Source: CAD feature listing. Evaluate the final solid. Frame: model axes, mm. Coordinates: 2 decimals unless noted, no trailing zeros. Write each loop counter-clockwise with the first axis right and the second up, starting at its lowest first coordinate (ties: lowest second). Pieces come first, ordered by that corner, then holes. Notation, with made-up numbers: (72.5, 70.25) -> (86.5, 70.25) arc R20 cw to (86.5, 109.25) -> close; hole circle Ø4 at (-15, 33.25). An arc over 180 degrees is marked (long way). Write item = value, one per line.
from build123d import *

# Parameters (mm, degrees)
F4_R     = 10.2299469816
F0_DEPTH = 127
F1_R     = 13.3830980952
F5_DEPTH = 25.4
F3_SIZE  = 10.16
F6_R     = 5.08


# Not quite as in the source:
# - a fillet or chamfer that OpenCascade refuses, or shapes differently, is made with other operations: its cross-section is extruded or revolved along the edge and cut away or added


with BuildPart() as f0:
    # F4 (on Top) → F0 (new body)
    with BuildSketch(Plane.XY):
        Circle(F4_R)
    extrude(amount=F0_DEPTH)

    # F1 (on face) → F5 (join)
    with BuildSketch(Plane.XY.offset(127)):
        Circle(F1_R)
    extrude(amount=F5_DEPTH)

    # F2: fillet of radius 5.08 on 1 edges, made by hand

    # F2_s1 → F2_t2 (revolve, cut)
    with BuildSketch(Plane.XZ):
        with BuildLine():
            ThreePointArc((13.3830980952, 131.7003886402), (12.5217941226, 128.870370296), (10.2299469816, 127))
            Line((10.2299469816, 127), (13.3830980952, 127))
            Line((13.3830980952, 127), (13.3830980952, 131.7003886402))
        make_face()
    revolve(axis=Axis((0, 0, 127), (0, 0, 1)), mode=Mode.SUBTRACT)

    # F3
    f3_edges = [f0.edges().sort_by_distance(p)[0] for p in [
        (-13.383098, 0, 152.4),
    ]]
    chamfer(f3_edges, length=F3_SIZE)

    # F6
    f6_edges = [f0.edges().sort_by_distance(p)[0] for p in [
        (-3.223098, 0, 152.4),
    ]]
    fillet(f6_edges, radius=F6_R)


solid = f0.part
1) Cut plane B-B, the plane z = 73. Output: boundary loops of the cut face in (x, y).
Answer block:
outline = circle Ø20.46 at (0, 0)
2) First-contact query: pin 1 Ø6 at (x, z) = (-4, 46) entering from +Y; pin 2 Ø3 at (x, z) = (-6.5, 16) entering from +Y; pin 3 Ø2 at (x, z) = (8, 73.5) entering from +Y; pin 4 Ø10 at (x, y) = (3.5, 5) entering from -Z. Flat tips, straight axial feed; report the tip coordinate or a pass-through.
Answer block:
pin_1 = 10.18
pin_2 = 8.92
pin_3 = 7.46
pin_4 = 0
3) Material intervals for probe 1 along Y at (x, z) = (-0.5, 50); probe 2 along Y at (x, z) = (-1.5, 72); probe 3 along X at (y, z) = (-7, 33.5), sorted ascending. Write a range as [from, to].
Answer block:
probe_1 = [-10.22, 10.22]
probe_2 = [-10.12, 10.12]
probe_3 = [-7.46, 7.46]
4) Cut plane A-A, the plane z = 136.5. Output: boundary loops of the cut face in (x, y), and give its area (3 significant figures).
Answer block:
outline = circle Ø26.77 at (0, 0)
area = 563 mm2
5) Pull-direction query (X, two-part tool) for faces 1 (the cylindrical face through (9.76, 3.07, 62.61)), 2 (the flat face through (0, 0, 0)); classes: +X half, -X half, draft (parallel to the pull), parting line (faces both ways), or undercut.
Answer block:
face_1 = parting line
face_2 = draft
